The model under review builds one solid part; all positions refer to its coordinate system, in mm. A direction names the side the tool comes from. Give positions to 0.01 mm unless a question says otherwise; leave off trailing zeros. Order: outer loops, then holes, each group sorted by start corner. A loop starts at its lowest first (then second) coordinate and runs counter-clockwise, first axis right, second up.
```python
from build123d import *

# Parameters (mm, degrees)
F1_DEPTH = 5


with BuildPart() as f1:
    # F0 (on Front) → F1 (new body)
    with BuildSketch(Plane.XZ):
        Polygon((71.416639, 25.993531), (59.670481, 21.718279), (58.219378, 48.851858), (48.643822, 40.817013), (38, 65.817931), (31.75, 54.992613), (13.197262, 74.845389), (11.026659, 62.535292), (-13.197262, 74.845389), (-11.026659, 62.535292), (-38, 65.817931), (-31.75, 54.992613), (-58.219378, 48.851858), (-48.643822, 40.817013), (-71.416639, 25.993531), (-59.670481, 21.718279), (-76, 0), (-63.5, 0), (-71.416639, -25.993531), (-59.670481, -21.718279), (-58.219378, -48.851858), (-48.643822, -40.817013), (-38, -65.817931), (-31.75, -54.992613), (-13.197262, -74.845389), (-11.026659, -62.535292), (13.197262, -74.845389), (11.026659, -62.535292), (38, -65.817931), (31.75, -54.992613), (58.219378, -48.851858), (48.643822, -40.817013), (71.416639, -25.993531), (59.670481, -21.718279), (76, 0), (63.5, 0), align=None)
        with BuildLine():
            ThreePointArc((3, 18.761663), (14.456832, 12.328828), (19, 0))
            ThreePointArc((19, 0), (-12.328828, -14.456832), (-3, 18.761663))
            Line((-3, 18.761663), (-3, 22))
            Line((-3, 22), (3, 22))
            Line((3, 22), (3, 18.761663))
        make_face(mode=Mode.SUBTRACT)
    extrude(amount=F1_DEPTH)


solid = f1.part
```
1. Draft analysis for pull direction X (two halves, no side actions). For faces 4 (the flat face through (-12.127, -2.465, -68.777)), 5 (the flat face through (-34.92, -2.46, 60.48)), 6 (the flat face through (12.127, -2.465, -68.777)), 7 (the flat face through (59.87, -2.46, -33.51)), state which applies: pulls with the +X half, pulls with the -X half, needs draft (parallel to the pull), parting line crosses it, or undercut.
2. Take a section at A-A (x = 0). Write out the cut boundary in (y, z), and give its area (3 significant figures).
3. Insertion check: pin 1 (1.5 mm diameter, centred on x = -70.5, y = -2.5, fed in from -Z); pin 2 (3 mm diameter, centred on y = -0.5, z = 11, fed in from +X); pin 3 (1 mm diameter, centred on y = -3.5, z = 20, fed in from +X). Each pin has a flat end and moves straight along its axis. Give the tip position at first contact, or say it passes through.
4. Take a section at C-C (z = 32). Write out the cut boundary in (x, y).
5. Take a section at B-B (z = -57). Write out the cut boundary in (x, y).
6. For faces 1 (the flat face through (67.4, -2.5, 12.8)), 2 (the flat face through (65.626, -2.465, 23.886)), 3 (the flat face through (-12.127, -2.465, 68.777)), list the 3-axis set-ups (+Z, -Z, +X, -X, +Y, -Y) from which the entire face can be reached by the end or side of a thin tool; tool diameter is ignored.
7. To check wall thickness, follow line 1 (Z direction, x = -36, y = -1.7); line 2 (Z direction, x = 0, y = -1.2); line 3 (X direction, y = -0.6, z = -66). State the ranges of each line that lie inside material, in increasing order.
Answer:
1. face 4: undercut
1. face 5: pulls with the -X half
1. face 6: undercut
1. face 7: pulls with the +X half
2. outline: (-5, -68.14) - (0, -68.14) - (0, -19) - (-5, -19) - close; (-5, 22) - (0, 22) - (0, 68.14) - (-5, 68.14) - close
2. area: 476 mm2
3. pin 1: stops at z = -25.93
3. pin 2: stops at x = 67.31
3. pin 3: stops at x = 69.74
4. outline: (-62.19, -5) - (59.12, -5) - (59.12, 0) - (-62.19, 0) - close
5. outline: (-41.75, -5) - (-32.91, -5) - (-32.91, 0) - (-41.75, 0) - close; (-29.87, -5) - (32.91, -5) - (32.91, 0) - (-29.87, 0) - close
6. face 1: +X, +Y, -Y
6. face 2: +Z, +Y, -Y
6. face 3: +Y, -Y
7. line 1: z = -62.35 to 54.01, 62.35 to 65.57
7. line 2: z = -68.14 to -19, 22 to 68.14
7. line 3: x = -21.46 to -11.64, -4.21 to 11.64
